Here's the drawing with two shaded views (mm, measured from the low corner). I have some questions. A direction names the side the tool comes from. Coordinates: 2 decimals unless noted, no trailing zeros. Write each loop counter-clockwise with the first axis right and the second up, starting at its lowest first coordinate (ties: lowest second). Pieces come first, ordered by that corner, then holes.
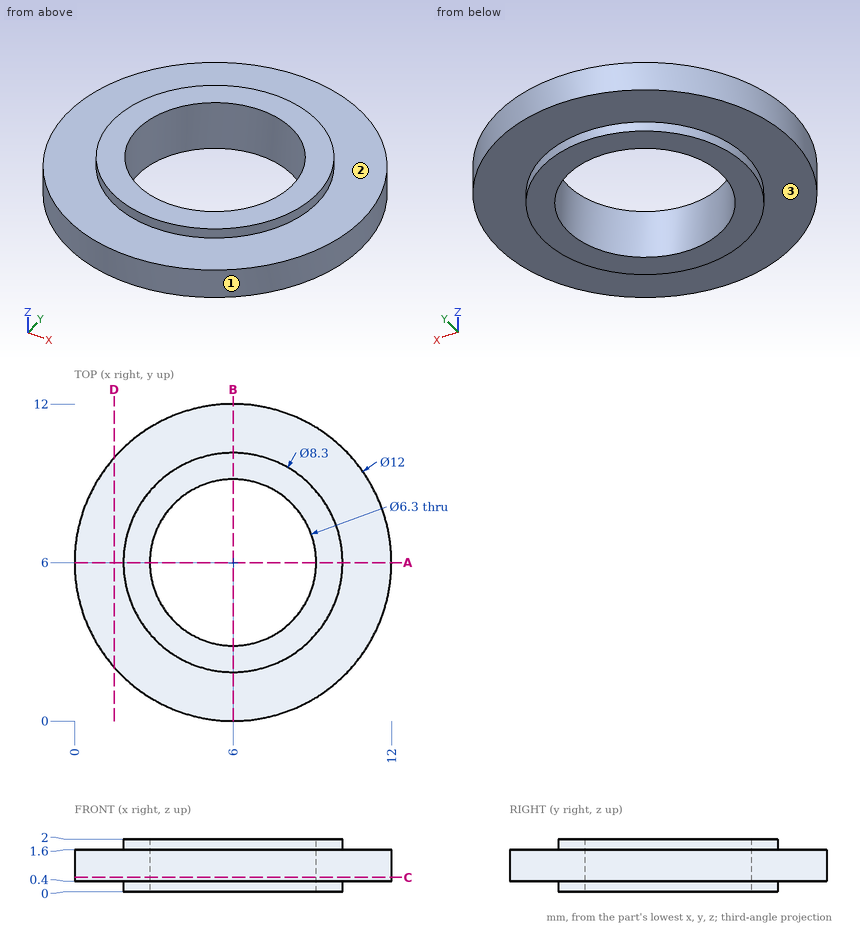
Item 1: I want a section at D-D, the plane x = 1.5. List the corners of the cut face in (y, z) for me.
Item 2: I want a section at A-A, the plane y = 6. List the corners of the cut face in (x, z) for me, then the cut area to 3 significant figures.
Item 3: I want a section at C-C, the plane z = 0.55. List the corners of the cut face in (x, y) for me.
Item 4: Will these pins go through, and if not, where does the flat tip stop? pin 1 Ø1 at (x, z) = (2.5, 1.5) entering from +Y; pin 2 Ø1 at (x, z) = (4, 1.5) entering from +Y.
Item 5: Which directions (+Z, -Z, +X, -X, +Y, -Y) give clear straight access to the entire face, cutting with the end or side of a thin tool? Please do the marked faces 1, 2 and 3.
Item 6: If I drill on line 1 along Y through (x, z) = (6, 0.7); line 2 along Z through (x, y) = (9.5, 3.5); line 3 along X through (y, z) = (5.5, 0.55), over which ranges is the centre line in solid material (lowest first)?
Taken from the geometry:
1. outline: (2.03, 0.4) - (9.97, 0.4) - (9.97, 1.6) - (2.03, 1.6) - close
2. outline: (0, 0.4) - (1.85, 0.4) - (1.85, 0) - (2.85, 0) - (2.85, 2) - (1.85, 2) - (1.85, 1.6) - (0, 1.6) - close; (9.15, 0) - (10.15, 0) - (10.15, 0.4) - (12, 0.4) - (12, 1.6) - (10.15, 1.6) - (10.15, 2) - (9.15, 2) - close
2. area: 8.44 mm2
3. outline: circle Ø12 at (6, 6); hole circle Ø6.3 at (6, 6)
4. pin 1: stops at y = 11.2
4. pin 2: stops at y = 11.81
5. face 1: +Z, -Z
5. face 2: +Z
5. face 3: -Z
6. line 1: y = 0 to 2.85, 9.15 to 12
6. line 2: z = 0.4 to 1.6
6. line 3: x = 0.02 to 2.89, 9.11 to 11.98
